```python
from build123d import *

# Parameters (mm, degrees)
SKETCH1_W           = 9
SKETCH1_H           = 8
BOSS_EXTRUDE1_DEPTH = 290
SKETCH2_W           = 20
SKETCH2_H           = 3
BOSS_EXTRUDE2_DEPTH = 40
SKETCH3_W           = 5
SKETCH3_H           = 4
CUT_EXTRUDE1_DEPTH  = 20


with BuildPart() as part:
    # Sketch1 → Boss-Extrude1 (new body)
    with BuildSketch(Plane.XY):
        Rectangle(SKETCH1_W, SKETCH1_H)
    extrude(amount=BOSS_EXTRUDE1_DEPTH)

    # Sketch2 → Boss-Extrude2 (add)
    with BuildSketch(Plane(origin=(4.5, 0, 0), x_dir=(0, 0, -1), z_dir=(1, 0, 0))):
        with Locations((-10, -2.5)):
            Rectangle(SKETCH2_W, SKETCH2_H)
    extrude(amount=BOSS_EXTRUDE2_DEPTH)

    # Sketch3 → Cut-Extrude1 (cut)
    with BuildSketch(Plane.XY.offset(290)):
        Rectangle(SKETCH3_W, SKETCH3_H)
    extrude(amount=-CUT_EXTRUDE1_DEPTH, mode=Mode.SUBTRACT)


solid = part.part
```
Could you check a few things on this model? Use its own coordinates, in mm. A direction names the side the tool comes from. Give positions to 0.01 mm unless a question says otherwise; leave off trailing zeros. Order: outer loops, then holes, each group sorted by start corner. A loop starts at its lowest first (then second) coordinate and runs counter-clockwise, first axis right, second up.
Q1. I'm going to push flat-ended pins straight in: P1, Ø3, axis at x = 18, y = 1, coming from the +Z side; P2, Ø2, axis at x = 1, y = -0.5, coming from the +Z side; P3, Ø4, axis at x = 27, y = -0.5, coming from the +Z side; P4, Ø2, axis at y = 1, z = 284.5, coming from the +X side. Where does each tip first touch, or does it pass through?
Q2. Suppose I cut it at D-D, the plane x = 39. Write out the boundary of the cut face in (y, z), and give its area (3 significant figures).
Q3. We'd pull the mould along X, two halves only. Please class faces 3 (the flat face through (-4.5, 0, 143)), 4 (the flat face through (0, -2, 280)), 5 (the flat face through (14, -2, 0)), 6 (the flat face through (0, 2, 280)): +X half, -X half, draft (parallel to the pull), parting line (faces both ways), or undercut.
Q4. Suppose I cut it at A-A, the plane y = 0.5. Write out the boundary of the cut face in (x, z), and give its area (3 significant figures).
Q5. If I drill on line 1 along Z through (x, y) = (40.5, -3); line 2 along X through (y, z) = (-0.25, 146); line 3 along Z through (x, y) = (0, 0.5), over which ranges is the centre line in solid material (lowest first)?
Q6. Suppose I cut it at B-B, the plane x = 0. Write out the boundary of the cut face in (y, z), and give its area (3 significant figures).
Q7. For faces 1 (the flat face through (0, 3, 290)), 2 (the flat face through (24, -1, 10)), which set-ups out of +Z, -Z, +X, -X, +Y, -Y let a thin tool reach every point of the face, with its end or its side?
Q8. Suppose I cut it at C-C, the plane z = 153.5. Write out the boundary of the cut face in (x, y), and give its area (3 significant figures).
Solution:
1. P1: passes through
1. P2: stops at z = 270
1. P3: stops at z = 20
1. P4: stops at x = 4.5
2. outline: (-4, 0) - (-1, 0) - (-1, 20) - (-4, 20) - close
2. area: 60.0 mm2
3. face 3: -X half
3. face 4: undercut
3. face 5: draft
3. face 6: undercut
4. outline: (-4.5, 0) - (4.5, 0) - (4.5, 290) - (2.5, 290) - (2.5, 270) - (-2.5, 270) - (-2.5, 290) - (-4.5, 290) - close
4. area: 2,510 mm2
5. line 1: z = 0 to 20
5. line 2: x = -4.5 to 4.5
5. line 3: z = 0 to 270
6. outline: (-4, 0) - (4, 0) - (4, 290) - (2, 290) - (2, 270) - (-2, 270) - (-2, 290) - (-4, 290) - close
6. area: 2,240 mm2
7. face 1: +Z, +X, -X, +Y, -Y
7. face 2: +Z, -Z, +X, +Y
8. outline: (-4.5, -4) - (4.5, -4) - (4.5, 4) - (-4.5, 4) - close
8. area: 72.0 mm2
